Can you work these out from the model? Positions are in its coordinate system, mm. A direction names the side the tool comes from. Coordinates: 2 decimals unless noted, no trailing zeros. Order: outer loops, then holes, each group sorted by start corner. A loop starts at its lowest first (then second) coordinate and runs counter-clockwise, first axis right, second up.
```python
from build123d import *

# Parameters (mm, degrees)
BOSS_EXTRUDE1_DEPTH = 57
SKETCH4_R           = 11
SKETCH4_R_2         = 2.5
CUT_EXTRUDE3_DEPTH  = 43
SKETCH5_W           = 73.1
SKETCH5_H           = 10
BOSS_EXTRUDE2_DEPTH = 77.1
SKETCH6_W           = 73.1
SKETCH6_H           = 10
BOSS_EXTRUDE3_DEPTH = 20
SKETCH8_W           = 73.1
SKETCH8_H           = 77.3
BOSS_EXTRUDE4_DEPTH = 10
SKETCH9_W           = 68.1
SKETCH9_H           = 57.3
CUT_EXTRUDE4_DEPTH  = 0.5


with BuildPart() as part:
    # Sketch1 → Boss-Extrude1 (new body)
    with BuildSketch(Plane.XY):
        Polygon((-34.05, 0), (34.05, 0), (34.05, -10), (29.05, -10), (-34.05, -10), (-39.05, -10), (-39.05, 57.3), (-34.05, 57.3), align=None)
    extrude(amount=BOSS_EXTRUDE1_DEPTH)

    # Sketch4 → Cut-Extrude3 (cut)
    with BuildSketch(Plane.ZY.offset(39.05)):
        with Locations(Location((28.5, 28.65, 0), (0, 0, 270))):
            Circle(SKETCH4_R)
        with Locations(Location((52.07, 52.22, 0), (0, 0, 270))):
            Circle(SKETCH4_R_2)
        with Locations(Location((4.93, 52.22, 0), (0, 0, 270))):
            Circle(SKETCH4_R_2)
        with Locations(Location((52.07, 5.08, 0), (0, 0, 270))):
            Circle(SKETCH4_R_2)
        with Locations(Location((4.93, 5.08, 0), (0, 0, 270))):
            Circle(SKETCH4_R_2)
    extrude(amount=-CUT_EXTRUDE3_DEPTH, mode=Mode.SUBTRACT)

    # Sketch5 → Boss-Extrude2 (add)
    with BuildSketch(Plane.XZ.offset(10)):
        with Locations((-2.5, 5)):
            Rectangle(SKETCH5_W, SKETCH5_H)
        with Locations((-2.5, 52)):
            Rectangle(SKETCH5_W, SKETCH5_H)
    extrude(amount=BOSS_EXTRUDE2_DEPTH)

    # Sketch6 → Boss-Extrude3 (add)
    with BuildSketch(Plane(origin=(0, 0, 0), x_dir=(-1, 0, 0), z_dir=(0, 0, -1))):
        with Locations((2.5, -82.1)):
            Rectangle(SKETCH6_W, SKETCH6_H)
    boss_extrude3 = extrude(amount=BOSS_EXTRUDE3_DEPTH)

    # Sketch8 → Boss-Extrude4 (add)
    with BuildSketch(Plane(origin=(0, 0, 0), x_dir=(-1, 0, 0), z_dir=(0, 0, -1))):
        with Locations((2.5, 18.65)):
            Rectangle(SKETCH8_W, SKETCH8_H)
    boss_extrude4 = extrude(amount=BOSS_EXTRUDE4_DEPTH)

    # Mirror2: Boss-Extrude4 across plane
    add(boss_extrude4.mirror(Plane.XY.offset(28.5)))

    # Mirror3: Boss-Extrude3 across plane
    add(boss_extrude3.mirror(Plane.XY.offset(28.5)))

    # Sketch9 → Cut-Extrude4 (cut)
    with BuildSketch(Plane(origin=(0, 0, 57), x_dir=(-1, 0, 0), z_dir=(0, 0, -1))):
        with Locations((0, 28.65)):
            Rectangle(SKETCH9_W, SKETCH9_H)
    cut_extrude4 = extrude(amount=-CUT_EXTRUDE4_DEPTH, mode=Mode.SUBTRACT)

    # Mirror4: Cut-Extrude4 across plane
    add(cut_extrude4.mirror(Plane.XY.offset(28.5)), mode=Mode.SUBTRACT)


solid = part.part
```
1. Please list where these lines run through material, in increasing order: probe 1 along Z at (x, y) = (-36.15, 52.22); probe 2 along Y at (x, z) = (-38, 52); probe 3 along Z at (x, y) = (-26, 10.5).
Completed:
probe 1: z = -10 to 2.43, 7.43 to 49.57, 54.57 to 67
probe 2: y = -87.1 to 2.58, 7.58 to 49.72, 54.72 to 57.3
probe 3: z = -10 to -0.5, 57.5 to 67
2. Imagine slicing it at A-A on y = 5.08. Please give me the cut outline in (x, z), then the cut area to 3 significant figures.
Completed:
outline: (-39.05, -10) - (34.05, -10) - (34.05, -0.5) - (-34.05, -0.5) - (-34.05, 2.43) - (-39.05, 2.43) - close; (-39.05, 7.43) - (-34.05, 7.43) - (-34.05, 49.57) - (-39.05, 49.57) - close; (-39.05, 54.57) - (-34.05, 54.57) - (-34.05, 57.5) - (34.05, 57.5) - (34.05, 67) - (-39.05, 67) - close
area: 1,630 mm2
3. On a 3-axis mill with a long thin cutter (end or side, diameter ignored), from which of +Z, -Z, +X, -X, +Y, -Y can I reach the whole of each face in a straight line? I mean faces 5 (the flat face through (-2, 19, 67)), 6 (the flat face through (0, 29, 57.5)), 7 (the flat face through (-3, -48, 0)), 8 (the flat face through (-3, -48, 47)), 9 (the flat face through (-2, 19, -10)). Say none if no direction works.
Completed:
face 5: +Z, +X, -X, +Y
face 6: +X, +Y
face 7: -Z, +X, -X
face 8: +X, -X, -Y
face 9: -Z, +X, -X, +Y
4. I'm going to push flat-ended pins straight in: pin 1 (1.5 mm diameter, centred on x = -21, y = -38, fed in from -Z); pin 2 (16 mm diameter, centred on x = -18.5, z = 71.5, fed in from +Y); pin 3 (8 mm diameter, centred on x = 15.5, y = -47.5, fed in from +Z); pin 4 (12 mm diameter, centred on x = 25.5, y = 19, fed in from +Z). Where does each tip first touch, or does it pass through?
Completed:
pin 1: stops at z = 0
pin 2: stops at y = 57.3
pin 3: stops at z = 57
pin 4: stops at z = 67
5. Thinking about a two-plate mould opening in Y: for faces 1 (the flat face through (-3, -10, 28)), 2 (the flat face through (0, 0, 29)), 3 (the flat face through (-2, -48, 57)), 4 (the flat face through (-2, -77.1, -10)), which applies, pulls with the +Y half, pulls with the -Y half, needs draft (parallel to the pull), parting line crosses it, or undercut?
Completed:
face 1: pulls with the -Y half
face 2: pulls with the +Y half
face 3: undercut
face 4: undercut
6. Imagine slicing it at C-C on y = -12.5. Please give me the cut outline in (x, z).
Completed:
outline: (-39.05, -10) - (34.05, -10) - (34.05, 10) - (-39.05, 10) - close; (-39.05, 47) - (34.05, 47) - (34.05, 67) - (-39.05, 67) - close
7. Imagine slicing it at B-B on z = 4.93. Please give me the cut outline in (x, y), then the cut area to 3 significant figures.
Completed:
outline: (-39.05, -87.1) - (34.05, -87.1) - (34.05, 0) - (-34.05, 0) - (-34.05, 2.58) - (-39.05, 2.58) - close; (-39.05, 7.58) - (-34.05, 7.58) - (-34.05, 49.72) - (-39.05, 49.72) - close; (-39.05, 54.72) - (-34.05, 54.72) - (-34.05, 57.3) - (-39.05, 57.3) - close
area: 6,600 mm2
8. Imagine slicing it at D-D on z = 28.5. Please give me the cut outline in (x, y).
Completed:
outline: (-39.05, -10) - (34.05, -10) - (34.05, 0) - (-34.05, 0) - (-34.05, 17.65) - (-39.05, 17.65) - close; (-39.05, 39.65) - (-34.05, 39.65) - (-34.05, 57.3) - (-39.05, 57.3) - close
